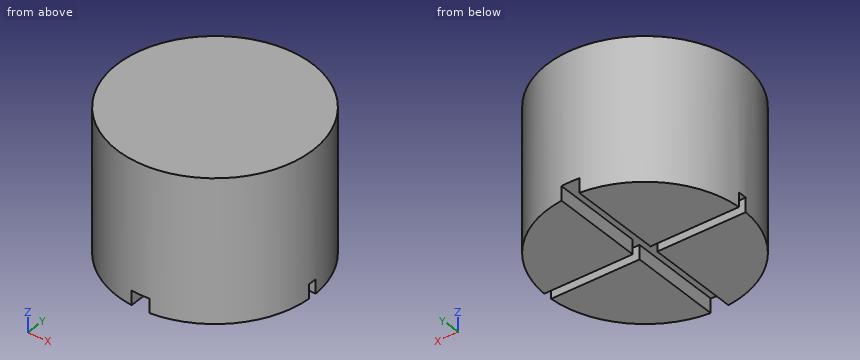
from build123d import *

# Parameters (mm, degrees)
SKETCH1_R           = 17.4625
BOSS_EXTRUDE1_DEPTH = 25.4
CUT_EXTRUDE1_DEPTH  = 2.54


with BuildPart() as part:
    # Sketch1 → Boss-Extrude1 (new body)
    with BuildSketch(Plane.XY):
        Circle(SKETCH1_R)
    extrude(amount=BOSS_EXTRUDE1_DEPTH)

    # Sketch2 → Cut-Extrude1 (cut)
    with BuildSketch(Plane(origin=(0, 0, 0), x_dir=(-1, 0, 0), z_dir=(0, 0, -1))):
        Polygon((1.5875, 0.79375), (23.225772956, 0.79375), (23.225772956, -0.79375), (1.5875, -0.79375), (1.5875, -19.542370193), (-1.5875, -19.542370193), (-1.5875, -0.79375), (-24.356135007, -0.79375), (-24.356135007, 0.79375), (-1.5875, 0.79375), (-1.5875, 20.58214549), (1.5875, 20.58214549), align=None)
    extrude(amount=-CUT_EXTRUDE1_DEPTH, mode=Mode.SUBTRACT)


solid = part.part
Geometry check sheet. Reference: the model listing, model coordinates, mm. Round coordinates to 2 decimals unless told otherwise and drop trailing zeros. Loops run counter-clockwise (first coordinate to the right, second up) from the corner with the lowest first, then second, coordinate; pieces in that order, holes last. Notation, with made-up numbers: (32, 53.5) -> (56, 53.5) arc R24 cw to (56, 71.5) -> close; hole circle Ø8 at (70.25, 74). An arc over 180 degrees is marked (long way). Answer as a JSON object with one key per item and string values. Group by question number.
Item 1: Cross-section at A-A, the plane y = 5. Record the cut outline in (x, z), plus the area to 3 significant figures.
Item 2: Cross-section at C-C, the plane z = 11.5. Record the cut outline in (x, y) (1 decimal).
Item 3: Depth check by flat-ended pin: pin 1 Ø8 at (x, z) = (-5, 7.5) entering from +Y; pin 2 Ø0.8 at (x, z) = (7.5, 1) entering from +Y; pin 3 Ø2 at (x, z) = (-6, 1) entering from +Y; pin 4 Ø17.5 at (x, y) = (-2.5, 1.5) entering from -Z. Enter the tip coordinate at first touch or a pass-through.
Item 4: Cross-section at B-B, the plane x = -13. Record the cut outline in (y, z), plus the area to 3 significant figures.
Item 5: Thickness scan on line 1 along Z through (x, y) = (-0.5, 5); line 2 along Y through (x, z) = (-11.5, 2.5); line 3 along X through (y, z) = (-9.5, 1.25). Record the ranges inside material, lowest first.
Item 6: Cross-section at D-D, the plane x = 0. Record the cut outline in (y, z), plus the area to 3 significant figures.
Determined:
{
 "1": {"outline": "(-16.73, 0) -> (-1.59, 0) -> (-1.59, 2.54) -> (1.59, 2.54) -> (1.59, 0) -> (16.73, 0) -> (16.73, 25.4) -> (-16.73, 25.4) -> close", "area": "842 mm²"},
 "2": {"outline": "circle Ø34.9 at (0, 0)"},
 "3": {"pin 1": "stops at y = 17.43", "pin 2": "stops at y = 15.95", "pin 3": "stops at y = 16.73", "pin 4": "stops at z = 0"},
 "4": {"outline": "(-11.66, 0) -> (-0.79, 0) -> (-0.79, 2.54) -> (0.79, 2.54) -> (0.79, 0) -> (11.66, 0) -> (11.66, 25.4) -> (-11.66, 25.4) -> close", "area": "588 mm²"},
 "5": {"line 1": "z = 2.54 to 25.4", "line 2": "y = -13.14 to -0.79, 0.79 to 13.14", "line 3": "x = -14.65 to -1.59, 1.59 to 14.65"},
 "6": {"outline": "(-17.46, 2.54) -> (17.46, 2.54) -> (17.46, 25.4) -> (-17.46, 25.4) -> close", "area": "798 mm²"}
}
